Geometry: final body of the model. Coordinates: model frame, mm. A direction names the side the tool comes from. Round coordinates to 2 decimals unless told otherwise and drop trailing zeros. Write each loop counter-clockwise with the first axis right and the second up, starting at its lowest first coordinate (ties: lowest second). Pieces come first, ordered by that corner, then holes. Notation, with made-up numbers: M 69,64.5 L 110,64.5 A18 ccw 110,97.5 Z; hole C 36,44.25 d9. An arc over 180 degrees is marked long. Answer as CSV lines item,"result". Start each with the question number.
Q1. Section query A-A on y = 10.75. Output: boundary loops of the cut face in (x, z), and give its area (3 significant figures).
Q2. Section query D-D on y = 0. Output: boundary loops of the cut face in (x, z), and give its area (3 significant figures).
Q3. Reachability of faces 1 (the flat face through (-9, 12.7, 0)), 2 (the cylindrical face through (-1.616, -7.278, -75.008)) from +Z, -Z, +X, -X, +Y, -Y: full face, straight path, thin tool, end or side. Return the list, or none.
Q4. Ray query, probe 1 along Z at (x, y) = (-13, 11.25); probe 2 along X at (y, z) = (0.5, -20.5); probe 3 along Z at (x, y) = (22.5, 2.25). Return the intervals inside material, ascending.
Q5. Section query C-C on z = -111.5. Output: boundary loops of the cut face in (x, y).
Q6. Section query B-B on x = 0. Output: boundary loops of the cut face in (y, z).
Q7. First-contact query: pin 1 (6 mm diameter, centred on y = -2.5, z = -68, fed in from +X); pin 2 (8 mm diameter, centred on x = -12, y = -6.5, fed in from -Z); pin 3 (6 mm diameter, centred on y = -2, z = -21.5, fed in from -X). Flat tips, straight axial feed; report the tip coordinate or a pass-through.
```python
from build123d import *

# Parameters (mm, degrees)
F1_DEPTH = 12.7
F2_R     = 7.455635
F3_DEPTH = 136.652
F4_R     = 5.167347
F5_R     = 3.066051
F6_R     = 26.453002


with BuildPart() as f1:
    # F0 (on Front) → F1 (new body, symmetric)
    with BuildSketch(Plane.XZ):
        Polygon((38.175546, -5.210182), (4.778824, 15.066399), (-38.175546, 15.066399), (-38.175546, -15.066399), (38.175546, -15.066399), align=None)
    extrude(amount=F1_DEPTH, both=True)

    # F2 (on Top) → F3 (join)
    with BuildSketch(Plane.XY):
        Circle(F2_R)
    extrude(amount=-F3_DEPTH)

    # F4
    f4_edges = [f1.edges().sort_by_distance(p)[0] for p in [
        (38.175546, 0, -5.210182),
    ]]
    fillet(f4_edges, radius=F4_R)

    # F5
    f5_edges = [f1.edges().sort_by_distance(p)[0] for p in [
        (38.175546, 0, -15.066399),
    ]]
    fillet(f5_edges, radius=F5_R)

    # F6
    f6_edges = [f1.edges().sort_by_distance(p)[0] for p in [
        (4.778824, 0, 15.066399),
    ]]
    fillet(f6_edges, radius=F6_R)


solid = f1.part
```
Entries:
1,outline,"M -38.18,-15.07 L 35.11,-15.07 A3.07 ccw 38.18,-12 L 38.18,-8.12 A5.17 ccw 35.69,-3.7 L 11.11,11.23 A26.45 ccw -2.62,15.07 L -38.18,15.07 Z"
1,area,"1,950 mm^2"
2,outline,"M -38.18,-15.07 L -7.46,-15.07 L -7.46,-136.65 L 7.46,-136.65 L 7.46,-15.07 L 35.11,-15.07 A3.07 ccw 38.18,-12 L 38.18,-8.12 A5.17 ccw 35.69,-3.7 L 11.11,11.23 A26.45 ccw -2.62,15.07 L -38.18,15.07 Z"
2,area,"3,770 mm^2"
3,face 1,"+Z, -Z, +X, -X, +Y"
3,face 2,"-Z"
4,probe 1,"z = -15.07 to 15.07"
4,probe 2,"x = -7.44 to 7.44"
4,probe 3,"z = -15.07 to 4.31"
5,outline,"C 0,0 d14.91"
6,outline,"M -12.7,-15.07 L -7.46,-15.07 L -7.46,-136.65 L 7.46,-136.65 L 7.46,-15.07 L 12.7,-15.07 L 12.7,14.94 L -12.7,14.94 Z"
7,pin 1,"stops at x = 7.46"
7,pin 2,"stops at z = -15.07"
7,pin 3,"stops at x = -7.46"
